Verification items for the finished model (mm, model axes). Coordinates: 2 decimals unless noted, no trailing zeros. Order: outer loops, then holes, each group sorted by start corner. A loop starts at its lowest first (then second) coordinate and runs counter-clockwise, first axis right, second up. Notation, with made-up numbers: M 78,19.25 L 122,19.25 A30 ccw 122,51.25 Z; hole C 1.5,6.25 d3. An arc over 180 degrees is marked long. Use one line per item in the form item = value. Start each with the question number.
```python
from build123d import *

# Parameters (mm, degrees)
BOSS_EXTRUDE1_DEPTH = 15


with BuildPart() as part:
    # Sketch1 → Boss-Extrude1 (new body)
    with BuildSketch(Plane.XY):
        with BuildLine():
            Line((-99.134442938, 21.769328519), (-98.817115398, 22.553238929))
            Line((-98.817115398, 22.553238929), (-98.754280528, 22.708463115))
            ThreePointArc((-98.754280528, 22.708463115), (-102.100537724, 23.60025606), (-105.54024369, 24.001696896))
            Line((-105.54024369, 24.001696896), (-105.54024369, 23.834302043))
            Line((-105.54024369, 23.834302043), (-105.533426583, 22.988627268))
            Line((-105.533426583, 22.988627268), (-105.531003444, 22.68803248))
            ThreePointArc((-105.531003444, 22.68803248), (-105.475765577, 22.551638114), (-105.342161912, 22.489955815))
            ThreePointArc((-105.342161912, 22.489955815), (-102.381968354, 22.126893501), (-99.495686711, 21.375935169))
            ThreePointArc((-99.495686711, 21.375935169), (-99.34876179, 21.384163954), (-99.247236895, 21.490687852))
            Line((-99.247236895, 21.490687852), (-99.134442938, 21.769328519))
        make_face()
    extrude(amount=-BOSS_EXTRUDE1_DEPTH)


solid = part.part
```
1. Depth check by flat-ended pin: P1, Ø1.5, axis at y = 22, z = -7.5, coming from the +X side; P2, Ø4, axis at x = -105, z = -8, coming from the -Y side. Enter the tip coordinate at first touch or a pass-through.
2. Cross-section at C-C on y = 23.6. Enter the section's corners in (x, z).
3. Cross-section at A-A on z = -9.5. Enter the section's corners in (x, y) (3 decimals).
4. Cross-section at B-B on x = -100. Enter the section's corners in (y, z), and give its area (3 significant figures).
5. Material ranges on line 1 along Y through (x, z) = (-99.5, -5.5); line 2 along Y through (x, z) = (-100.25, -5.5); line 3 along X through (y, z) = (22.6, -2.5), recorded low to high.
Final values:
q1.P1 = -98.75
q1.P2 = 22.24
q2.outline = M -105.54,-15 L -102.1,-15 L -102.1,0 L -105.54,0 Z
q3.outline = M -105.54,23.834 L -105.531,22.688 A0.2 ccw -105.342,22.49 A22.525 cw -99.496,21.376 A0.2 ccw -99.247,21.491 L -98.754,22.708 A24.025 ccw -105.54,24.002 Z
q4.outline = M 21.54,-15 L 23.1,-15 L 23.1,0 L 21.54,0 Z
q4.area = 23.5 mm2
q5.line_1 = 21.38 to 22.95
q5.line_2 = 21.61 to 23.17
q5.line_3 = -105.51 to -98.8
